Here's how the part is built. I have some questions about the finished solid (model axes, mm). Round coordinates to 2 decimals unless told otherwise and drop trailing zeros. Order: outer loops, then holes, each group sorted by start corner. A loop starts at its lowest first (then second) coordinate and runs counter-clockwise, first axis right, second up. Notation, with made-up numbers: M 9,-1.75 L 55,-1.75 A15 cw 55,25.25 Z; hole C 83,89.5 d3. An arc over 180 degrees is marked long. Write item = value, one per line. Start each with the question number.
Item 1: I want a section at C-C, the plane z = 5. State how many separate pieces and enclosed holes the cut face has, plus the area to 3 significant figures.
Item 2: Please list where these lines run through material, in increasing order: L1, parallel to Y at x = 0, z = 3 (3 decimals); L2, parallel to X at y = 27, z = 6; L3, parallel to Y at x = 38, z = 4.25.
Item 3: We'd pull the mould along Y, two halves only. Please class faces 1 (the face through (28.406, 24.124, 3.131)), 2 (the face through (-11.012, -49.592, 1.878)), 3 (the face through (-1, 1, 6.35)), 4 (the face through (34.93, 0.14, 3.13)): pulls with the +Y half, pulls with the -Y half, needs draft (parallel to the pull), parting line crosses it, or undercut.
Item 4: I'm going to push flat-ended pins straight in: P1, Ø2, axis at y = -23.5, z = 3.5, coming from the -X side; P2, Ø1, axis at x = -16.5, z = 4.5, coming from the -Y side. Where does each tip first touch, or does it pass through?
Item 5: I want a section at A-A, the plane x = 0. List the corners of the cut face in (y, z) for me (3 decimals), plus the area to 3 significant figures.
```python
from build123d import *

# Parameters (mm, degrees)
F0_R     = 50.8
F0_R_2   = 3.175
F1_DEPTH = 6.35
F10_R    = 2.54


# Not quite as in the source:
# - the program builds the solid bodies; features that only make, move or delete a surface that nothing else refers to are left out


with BuildPart() as f1:
    # F0 (on Top) → F1 (new body)
    with BuildSketch(Plane.XY):
        Circle(F0_R)
        with Locations((-26.9407683632, -26.9407683632)):
            Circle(F0_R_2, mode=Mode.SUBTRACT)
        with Locations((0, -38.1)):
            Circle(F0_R_2, mode=Mode.SUBTRACT)
        with Locations((-38.1, 0)):
            Circle(F0_R_2, mode=Mode.SUBTRACT)
        with Locations((26.9407683632, -26.9407683632)):
            Circle(F0_R_2, mode=Mode.SUBTRACT)
        with Locations((38.1, 0)):
            Circle(F0_R_2, mode=Mode.SUBTRACT)
        with Locations((-26.9407683632, 26.9407683632)):
            Circle(F0_R_2, mode=Mode.SUBTRACT)
        with Locations((0, 38.1)):
            Circle(F0_R_2, mode=Mode.SUBTRACT)
        with Locations((26.9407683632, 26.9407683632)):
            Circle(F0_R_2, mode=Mode.SUBTRACT)
    extrude(amount=F1_DEPTH)

    # F10
    f10_edges = [f1.edges().sort_by_distance(p)[0] for p in [
        (-50.8, 0, 6.35),
    ]]
    fillet(f10_edges, radius=F10_R)


solid = f1.part
```
Filled in:
q1.separate_pieces = 1
q1.enclosed_holes = 8
q1.area = 7,760 mm^2
q2.L1 = -50.8 to -41.275, -34.925 to 34.925, 41.275 to 50.8
q2.L2 = -41.54 to -30.12, -23.77 to 23.77, 30.12 to 41.54
q2.L3 = -33.66 to -3.17, 3.17 to 33.66
q3.face_1 = undercut
q3.face_2 = parting line crosses it
q3.face_3 = needs draft
q3.face_4 = undercut
q4.P1 = -45.55
q4.P2 = -48.15
q5.outline = M -50.8,0 L -41.275,0 L -41.275,6.35 L -48.26,6.35 A2.54 ccw -50.8,3.81 Z; M -34.925,0 L 34.925,0 L 34.925,6.35 L -34.925,6.35 Z; M 41.275,0 L 50.8,0 L 50.8,3.81 A2.54 ccw 48.26,6.35 L 41.275,6.35 Z
q5.area = 562 mm^2
